Source: CAD feature listing. Evaluate the final solid. Frame: model axes, mm. Face numbers are marked on the shaded views. Round coordinates to 2 decimals unless told otherwise and drop trailing zeros. Order: outer loops, then holes, each group sorted by start corner. A loop starts at its lowest first (then second) coordinate and runs counter-clockwise, first axis right, second up. Notation, with made-up numbers: (61.25, -25.75) -> (80.25, -25.75) arc R33 cw to (80.25, 10.25) -> close; hole circle Ø3 at (47.25, 69.25). An arc over 180 degrees is marked (long way). Answer as CSV lines item,"result". Start each with the question number.
(1) Section query C-C (y = 1.05). Count the separate pieces of the cut face and the enclosed holes in it, plus the area to 3 significant figures.
(2) Pull-direction query (Z, two-part tool) for the marked faces 1 and 2; classes: +Z half, -Z half, draft (parallel to the pull), parting line (faces both ways), or undercut.
(3) Section query A-A (z = 9). Output: boundary loops of the cut face in (x, y).
(4) Section query B-B (x = 9.5). Output: boundary loops of the cut face in (y, z).
(5) Line query: line 1 along X through (y, z) = (1.8, -10.5); line 2 along Z through (x, y) = (-6.5, 0.2); line 3 along Z through (x, y) = (16, 1.6). Output: solid intervals per line, ascending. Write a range as from..to.
(6) Contact query for flat-ended pins moving along their axis: P1, Ø1.2, axis at x = 21, z = -22.5, coming from the +Y side; P2, Ø4, axis at x = 21, z = 6.5, coming from the -Y side. Output: stop coordinate, or through.
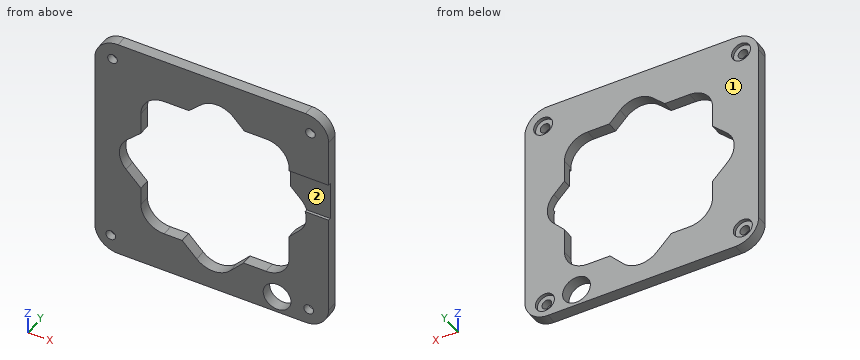
```python
from build123d import *

# Parameters (mm, degrees)
EXTRUDE_1_DEPTH      = 2.4
SKETCH_2_R           = 1.05000254
CUT_EXTRUDE_1_DEPTH  = 10
CUT_EXTRUDE_8_DEPTH  = 3.4
SKETCH_4_R           = 2.05
CUT_EXTRUDE_9_DEPTH  = 0.73
SKETCH_5_R           = 3
CUT_EXTRUDE_10_DEPTH = 3.4
SKETCH_6_W           = 27.234219955
SKETCH_6_H           = 8.445318751
CUT_EXTRUDE_12_DEPTH = 0.6


with BuildPart() as part:
    # 草图1 → 凸台-拉伸1 (new body)
    with BuildSketch(Plane(origin=(0, 0, 0), x_dir=(1, 0, 0), z_dir=(0, 1, 0))):
        with BuildLine():
            Line((-20.25, 25.25), (20.25, 25.25))
            ThreePointArc((20.25, 25.25), (23.785533906, 23.785533906), (25.25, 20.25))
            Line((25.25, 20.25), (25.25, -20.25))
            ThreePointArc((25.25, -20.25), (23.785533906, -23.785533906), (20.25, -25.25))
            Line((20.25, -25.25), (-20.25, -25.25))
            ThreePointArc((-20.25, -25.25), (-23.785533906, -23.785533906), (-25.25, -20.25))
            Line((-25.25, -20.25), (-25.25, 20.25))
            ThreePointArc((-25.25, 20.25), (-23.785533906, 23.785533906), (-20.25, 25.25))
        make_face()
    extrude(amount=EXTRUDE_1_DEPTH)

    # 草图2 → 切除-拉伸1 (cut)
    with BuildSketch(Plane(origin=(0, 2.4, 0), x_dir=(1, 0, 0), z_dir=(0, 1, 0))):
        with Locations((21.308392177, -20.927391415)):
            Circle(SKETCH_2_R)
        with Locations((-21.452692405, -21.308392177)):
            Circle(SKETCH_2_R)
        with Locations((-21.833693167, 21.452692405)):
            Circle(SKETCH_2_R)
        with Locations((20.927391415, 21.833693167)):
            Circle(SKETCH_2_R)
    extrude(amount=-CUT_EXTRUDE_1_DEPTH, mode=Mode.SUBTRACT)

    # 草图3 → 切除-拉伸8 (cut, through all)
    with BuildSketch(Plane(origin=(0, 2.4, 0), x_dir=(1, 0, 0), z_dir=(0, 1, 0))):
        with BuildLine():
            Line((-18.515650574, 4.18369185), (-15.3, 7.427416998))
            Line((-15.3, 7.427416998), (-15.3, 11.4))
            ThreePointArc((-15.3, 11.4), (-13.835533906, 14.935533906), (-10.3, 16.4))
            Line((-10.3, 16.4), (-6.40507507, 16.4))
            Line((-6.40507507, 16.4), (-3.244074851, 19.588597663))
            ThreePointArc((-3.244074851, 19.588597663), (0.369210969, 21.068073973), (3.944434556, 19.49885096))
            Line((3.944434556, 19.49885096), (6.866728136, 16.4))
            Line((6.866728136, 16.4), (11.7, 16.4))
            ThreePointArc((11.7, 16.4), (15.235533906, 14.935533906), (16.7, 11.4))
            Line((16.7, 11.4), (16.7, 5.972627416))
            Line((16.7, 5.972627416), (19.047343924, 3.483463075))
            ThreePointArc((19.047343924, 3.483463075), (20.409425455, 0.000538557), (18.974455547, -3.452994511))
            Line((18.974455547, -3.452994511), (16.7, -5.765519402))
            Line((16.7, -5.765519402), (16.7, -10.6))
            ThreePointArc((16.7, -10.6), (15.235533906, -14.135533906), (11.7, -15.6))
            Line((11.7, -15.6), (7.027416998, -15.6))
            Line((7.027416998, -15.6), (4.702011711, -17.964327417))
            ThreePointArc((4.702011711, -17.964327417), (1.236457236, -19.457273038), (-2.285597178, -18.102988303))
            Line((-2.285597178, -18.102988303), (-4.950834187, -15.6))
            Line((-4.950834187, -15.6), (-10.3, -15.6))
            ThreePointArc((-10.3, -15.6), (-13.835533906, -14.135533906), (-15.3, -10.6))
            Line((-15.3, -10.6), (-15.3, -5.880848985))
            Line((-15.3, -5.880848985), (-18.387638433, -2.981173325))
            ThreePointArc((-18.387638433, -2.981173325), (-19.963985761, 0.57423879), (-18.515650574, 4.18369185))
        make_face()
    extrude(amount=-CUT_EXTRUDE_8_DEPTH, mode=Mode.SUBTRACT)

    # 草图4 → 切除-拉伸9 (cut)
    with BuildSketch(Plane(origin=(0, 2.4, 0), x_dir=(1, 0, 0), z_dir=(0, 1, 0))):
        with Locations((-21.833693167, 21.452692405)):
            Circle(SKETCH_4_R)
        with Locations((20.927391415, 21.833693167)):
            Circle(SKETCH_4_R)
        with Locations((21.308392177, -20.927391415)):
            Circle(SKETCH_4_R)
        with Locations((-21.452692405, -21.308392177)):
            Circle(SKETCH_4_R)
    extrude(amount=-CUT_EXTRUDE_9_DEPTH, mode=Mode.SUBTRACT)

    # 草图5 → 切除-拉伸10 (cut, through all)
    with BuildSketch(Plane(origin=(0, 2.4, 0), x_dir=(1, 0, 0), z_dir=(0, 1, 0))):
        with Locations((14.107378715, 21.590614681)):
            Circle(SKETCH_5_R)
    extrude(amount=-CUT_EXTRUDE_10_DEPTH, mode=Mode.SUBTRACT)

    # 草图6 → 切除-拉伸12 (cut)
    with BuildSketch(Plane.XZ):
        with Locations((26.071380204, 5.725361951)):
            Rectangle(SKETCH_6_W, SKETCH_6_H)
    extrude(amount=-CUT_EXTRUDE_12_DEPTH, mode=Mode.SUBTRACT)


solid = part.part
```
Answer block:
1,separate pieces,"1"
1,enclosed holes,"6"
1,area,"1,350 mm2"
2,face 1,"draft"
2,face 2,"undercut"
3,outline,"(-25.25, 0) -> (-15.3, 0) -> (-15.3, 2.4) -> (-25.25, 2.4) -> close; (16.7, 0.6) -> (25.25, 0.6) -> (25.25, 2.4) -> (16.7, 2.4) -> close"
4,outline,"(0, -25.25) -> (2.4, -25.25) -> (2.4, -16.4) -> (0, -16.4) -> close; (0, 15.6) -> (2.4, 15.6) -> (2.4, 25.25) -> (0, 25.25) -> close"
5,line 1,"-25.25..-15.3, 16.7..25.25"
5,line 2,"-25.25..-16.4, 15.6..25.25"
5,line 3,"-25.25..-23.92, -19.26..-13.95, 13.15..25.25"
6,P1,"y = 1.67"
6,P2,"y = 0.6"
